For this review, take the finished solid that the model builds, in its own axes (mm). Give positions to 0.01 mm unless a question says otherwise; leave off trailing zeros. Loops run counter-clockwise (first coordinate to the right, second up) from the corner with the lowest first, then second, coordinate; pieces in that order, holes last.
Autodesk Inventor part; units mm, degrees
ref_plane "YZ Plane" through (0, 0, 0) normal (1, 0, 0) x (0, 1, 0)
ref_plane "XZ Plane" through (0, 0, 0) normal (0, 1, 0) x (-1, 0, 0)
ref_plane "XY Plane" through (0, 0, 0) normal (0, 0, 1) x (1, 0, 0)
sketch "스케치3" plane through (0, 0, 0) normal (0, 0, 1) x (1, 0, 0)
  line L0 (0, 0) -> (1.15, 0)
  line L1 (1.15, 0) -> (1.15, -0.5)
  line L2 (1.15, -0.5) -> (0.8, -0.5)
  line L3 (0.8, -0.5) -> (0.8, -14.5)
  line L4 (0.8, -14.5) -> (0, -14.5)
  line L5 (0, -14.5) -> (0, 0)
  dimension "d13" = 1.15
  dimension "d14" = 0.5
  dimension "d15" = 14
  dimension "d16" = 0.8
revolve "회전2" add sketch "스케치3" angle 360 about axis through (0, -14.5, 0) along (0, 1, 0)
thread "스레드2"
sketch "스케치4" plane through (0, 0, 0) normal (0, 1, 0) x (1, 0, 0)
  line L0 (-0.15, -0.8) -> (0.15, -0.8)
  line L1 (0.15, -0.8) -> (0.15, 0.8)
  line L2 (0.15, 0.8) -> (-0.15, 0.8)
  line L3 (-0.15, 0.8) -> (-0.15, -0.8)
  line L4 (-0.15, -0.8) -> (0.15, 0.8) construction
  line L5 (0.15, -0.8) -> (-0.15, 0.8) construction
  line L6 (0.8, -0.15) -> (-0.8, -0.15)
  line L7 (-0.8, -0.15) -> (-0.8, 0.15)
  line L8 (-0.8, 0.15) -> (0.8, 0.15)
  line L9 (0.8, 0.15) -> (0.8, -0.15)
  circle A0 centre (0, 0) radius 0.8
  line L10 (0.8, -0.15) -> (-0.8, 0.15) construction
  line L11 (-0.8, -0.15) -> (0.8, 0.15) construction
  dimension "d21" = 0.3
  dimension "d22" = 1.6
  dimension "d23" = 1.6
  dimension "d24" = 0.3
extrude "돌출2" cut sketch "스케치4" against normal blind 0.3 contours L3 A0 L0 | A0 L1 L0 | A0 L3 L6 L1 | L6 A0 L8 L3 | L3 L8 L1 L6 | L6 L7 A0 | L1 L8 A0 L6 | A0 L9 L6 | L3 A0 L1 L8 | L7 L8 A0 | A0 L8 L9 | L3 L2 A0 | A0 L2 L1
properties part number "Screw"
Q1. For pin 1 Ø0.8 at (x, z) = (0, -0.5) entering from +Y, flat-tipped, find the tip position at first contact; note if it passes through.
Answers:
pin 1: stops at y = 0
Q2. Mouldability with a two-part tool opening along Z and no side actions: class faces 1 (the flat face through (0, -0.3, 0)), 2 (the cylindrical face through (-0.91, -0.25, -0.7)), 3 (the flat face through (0, -14.5, 0)) as +Z half, -Z half, draft (parallel to the pull), parting line (faces both ways), or undercut.
Answers:
face 1: undercut
face 2: parting line
face 3: draft
Q3. Consider section B-B on x = 0. Give the boundary of the cut face in (y, z).
Answers:
outline: (-14.5, -0.8) - (-0.5, -0.8) - (-0.5, -1.15) - (0, -1.15) - (0, -0.8) - (-0.3, -0.8) - (-0.3, 0.8) - (0, 0.8) - (0, 1.15) - (-0.5, 1.15) - (-0.5, 0.8) - (-14.5, 0.8) - close
Q4. Consider section A-A on z = 0. Give the boundary of the cut face in (x, y).
Answers:
outline: (-1.15, -0.5) - (-0.8, -0.5) - (-0.8, -14.5) - (0.8, -14.5) - (0.8, -0.5) - (1.15, -0.5) - (1.15, 0) - (0.8, 0) - (0.8, -0.3) - (-0.8, -0.3) - (-0.8, 0) - (-1.15, 0) - close
Q5. Consider section C-C on y = -2.5. Give the boundary of the cut face in (x, z).
Answers:
outline: circle Ø1.6 at (0, 0)
Q6. For probe 1 along Z at (x, y) = (0.05, -10.25); probe 2 along Y at (x, z) = (0.6, -0.05); probe 3 along Y at (x, z) = (0.4, 0.75), list the stretches that pass through material, from the lowest coordinate up.
Answers:
probe 1: z = -0.8 to 0.8
probe 2: y = -14.5 to -0.3
probe 3: y = -0.5 to 0
